Can you work these out from the model? Positions are in its coordinate system, mm. Round coordinates to 2 decimals unless told otherwise and drop trailing zeros. Loops run counter-clockwise (first coordinate to the right, second up) from the corner with the lowest first, then second, coordinate; pieces in that order, holes last. Notation, with made-up numbers: (65, -35.5) -> (111, -35.5) arc R28 cw to (111, -2.5) -> close; hole circle Ø4 at (4, -22.5). An arc over 180 degrees is marked (long way). Write item = value, one per line.
from build123d import *

# Parameters (mm, degrees)
BOSS_EXTRUDE1_DEPTH = 800


with BuildPart() as part:
    # Sketch1 → Boss-Extrude1 (new body)
    with BuildSketch(Plane(origin=(0, 0, 0), x_dir=(1, 0, 0), z_dir=(0, 1, 0))):
        with BuildLine():
            Line((-3.25, -5.04356025), (-6.15, -11.2))
            Line((-6.15, -11.2), (-6.15, -18.2))
            Line((-6.15, -18.2), (-15, -18.2))
            Line((-15, -18.2), (-15, -22.2))
            Line((-15, -22.2), (15, -22.2))
            Line((15, -22.2), (15, -18.2))
            Line((15, -18.2), (6.15, -18.2))
            Line((6.15, -18.2), (6.15, -11.2))
            Line((6.15, -11.2), (3.25, -5.04356025))
            ThreePointArc((3.25, -5.04356025), (0, 6), (-3.25, -5.04356025))
        make_face()
    extrude(amount=BOSS_EXTRUDE1_DEPTH)


solid = part.part
1. I'm going to push flat-ended pins straight in: pin 1 (5 mm diameter, centred on x = -12, y = 179, fed in from -Z); pin 2 (5.5 mm diameter, centred on y = 409.5, z = 15, fed in from +X); pin 3 (2 mm diameter, centred on y = 223, z = 1, fed in from +X). Where does each tip first touch, or does it pass through?
Entries:
pin_1 = 18.2
pin_2 = 6.15
pin_3 = 6
2. Suppose I cut it at A-A, the plane y = 442. List the corners of the cut face in (x, z) for me.
Entries:
outline = (-15, 18.2) -> (-6.15, 18.2) -> (-6.15, 11.2) -> (-3.25, 5.04) arc R6 ccw (long way) to (3.25, 5.04) -> (6.15, 11.2) -> (6.15, 18.2) -> (15, 18.2) -> (15, 22.2) -> (-15, 22.2) -> close
3. I need wall thicknesses on line 1 (Z direction, x = -12.5, y = 287); line 2 (X direction, y = 407, z = 13.75); line 3 (Z direction, x = 4, y = 35). Which ranges of each line are inside material? Lowest first, please. Write a range as [from, to].
Entries:
line_1 = [18.2, 22.2]
line_2 = [-6.15, 6.15]
line_3 = [-4.47, 4.47], [6.64, 22.2]
4. Suppose I cut it at B-B, the plane z = 0. List the corners of the cut face in (x, y) for me.
Entries:
outline = (-6, 0) -> (6, 0) -> (6, 800) -> (-6, 800) -> close
